from build123d import *

# Parameters (mm, degrees)
F0_W     = 10
F0_H     = 10
F1_DEPTH = 24
F3_D     = 3.6
F4_DEPTH = 10
F5_W     = 24
F5_H     = 4.0339039266
F6_DEPTH = 6.5
F7_DEPTH = 1.5


with BuildPart() as f1:
    # F0 (on Front) → F1 (new body)
    with BuildSketch(Plane.XZ):
        Rectangle(F0_W, F0_H)
    extrude(amount=F1_DEPTH)

    # F3 (through all)
    with Locations(Plane(origin=(-5, 0, 0), x_dir=(0, -1, 0), z_dir=(-1, 0, 0))):
        with Locations((12, 0)):
            Hole(F3_D / 2)

    # F4 (add): a face of the model
    f4_faces = [f1.faces().sort_by_distance(p)[0] for p in [
        (0, -12, -5),
    ]]
    extrude(f4_faces, amount=F4_DEPTH)

    # F5 (on face) → F6 (join)
    with BuildSketch(Plane(origin=(-5, 0, 0), x_dir=(0, -1, 0), z_dir=(-1, 0, 0))):
        with Locations((12, -12.9830480367)):
            Rectangle(F5_W, F5_H)
    extrude(amount=F6_DEPTH)

    # F7 (add): a face of the model
    f7_faces = [f1.faces().sort_by_distance(p)[0] for p in [
        (-11.5, -12, -12.9830480367),
    ]]
    extrude(f7_faces, amount=F7_DEPTH)


solid = f1.part
Here's how the part is built. I have some questions about the finished solid (model axes, mm). A direction names the side the tool comes from. Coordinates: 2 decimals unless noted, no trailing zeros. Order: outer loops, then holes, each group sorted by start corner. A loop starts at its lowest first (then second) coordinate and runs counter-clockwise, first axis right, second up. Notation, with made-up numbers: M -15.75,87.5 L -0.75,87.5 A16 cw -0.75,118.5 Z; hole C 73,-23 d2. An arc over 180 degrees is marked long. Answer as CSV lines item,"result". Start each with the question number.
1. For pin 1 (8 mm diameter, centred on y = -9.5, z = -5, fed in from -X); pin 2 (2.5 mm diameter, centred on x = -8.5, y = -8.5, fed in from +Z); pin 3 (2 mm diameter, centred on y = -12, z = 0, fed in from -X); pin 4 (12 mm diameter, centred on y = -2.5, z = -10.5, fed in from -X), each with a flat end and sliding along its axis, tell me the tip position at first contact or that it passes through.
2. On a 3-axis mill with a long thin cutter (end or side, diameter ignored), from which of +Z, -Z, +X, -X, +Y, -Y can I reach the whole of each face in a straight line? I mean faces 1 (the flat face through (-5, -12, -3)), 2 (the flat face through (-13, -12, -13)). Say none if no direction works.
3. I want a section at A-A, the plane y = -12. Write out the boundary of the cut face in (x, z).
4. I want a section at B-B, the plane z = 0. Write out the boundary of the cut face in (x, y).
5. I want a section at D-D, the plane x = -9. Write out the boundary of the cut face in (y, z), and give its area (3 significant figures).
6. We'd pull the mould along Z, two halves only. Please class faces 3 (the flat face through (0, -12, 5)), 4 (the flat face through (-2, -24, -7)), 5 (the cylindrical face through (0.07, -13.8, 0.08)): released by +Z, released by -Z, zero draft, split by the parting line, or undercut.
7. I need wall thicknesses on line 1 (Z direction, x = -2, y = -12); line 2 (X direction, y = -17, z = 2); line 3 (Z direction, x = -8, y = -11.25). Which ranges of each line are inside material? Lowest first, please. Write a range as [from, to].
8. I want a section at C-C, the plane x = 2.5. Write out the boundary of the cut face in (y, z).
Recorded:
1,pin 1,"stops at x = -5"
1,pin 2,"stops at z = -10.97"
1,pin 3,"passes through"
1,pin 4,"stops at x = -13"
2,face 1,"+Z, -X, +Y, -Y"
2,face 2,"+Z, -Z, -X, +Y, -Y"
3,outline,"M -13,-15 L 5,-15 L 5,-1.8 L -5,-1.8 L -5,-10.97 L -13,-10.97 Z; M -5,1.8 L 5,1.8 L 5,5 L -5,5 Z"
4,outline,"M -5,-24 L 5,-24 L 5,-13.8 L -5,-13.8 Z; M -5,-10.2 L 5,-10.2 L 5,0 L -5,0 Z"
5,outline,"M -24,-15 L 0,-15 L 0,-10.97 L -24,-10.97 Z"
5,area,"96.8 mm2"
6,face 3,"released by +Z"
6,face 4,"zero draft"
6,face 5,"undercut"
7,line 1,"z = [-15, -1.8], [1.8, 5]"
7,line 2,"x = [-5, 5]"
7,line 3,"z = [-15, -10.97]"
8,outline,"M -24,-15 L 0,-15 L 0,5 L -24,5 Z; hole C -12,0 d3.6"
